For this review, take the finished solid that the model builds, in its own axes (mm). A direction names the side the tool comes from. Round coordinates to 2 decimals unless told otherwise and drop trailing zeros. Write each loop counter-clockwise with the first axis right and the second up, starting at its lowest first coordinate (ties: lowest second). Pieces come first, ordered by that corner, then holes.
Solid Edge part; units mm, degrees
sketch "Sketch1" plane through (0, 0, 0) normal (0, -1, 0) x (1, 0, 0)
  circle A0 centre (0, 0) radius 4.5
extrude "Protrusion1" add sketch "Sketch1" against normal blind 170
hole "Hole_1" at (0, 3, 0) direction (-1, 0, 0) diameter 3 end up to next
hole "Hole_4" at (0, 164, 0) direction (1, 0, 0) diameter 7.94 end up to next
(1) We need section C-C, the plane y = 3. Give the boundary of the cut face in (x, z), and give its area (3 significant figures).
Geometry check:
outline: (-4.24, -1.5) arc R4.5 ccw (long way) to (-4.24, 1.5) - (0, 1.5) - (0, -1.5) - close
area: 50.4 mm2
(2) We need section D-D, the plane y = 164. Give the boundary of the cut face in (x, z), and give its area (3 significant figures).
Geometry check:
outline: (0, -3.97) - (0, 3.97) - (2.12, 3.97) arc R4.5 ccw (long way) to (2.12, -3.97) - close
area: 33.3 mm2
(3) We need section B-B, the plane y = 114. Give the boundary of the cut face in (x, z), and give its area (3 significant figures).
Geometry check:
outline: circle Ø9 at (0, 0)
area: 63.6 mm2
(4) We need section A-A, the plane z = 0. Give the boundary of the cut face in (x, y), and give its area (3 significant figures).
Geometry check:
outline: (-4.5, 0) - (4.5, 0) - (4.5, 160.03) - (0, 160.03) - (0, 167.97) - (4.5, 167.97) - (4.5, 170) - (-4.5, 170) - (-4.5, 4.5) - (0, 4.5) - (0, 1.5) - (-4.5, 1.5) - close
area: 1,480 mm2
(5) For pin 1 Ø4 at (y, z) = (163.5, -0.5) entering from +X; pin 2 Ø3 at (x, y) = (3, 104) entering from +Z; pin 3 Ø5 at (x, y) = (3, 107.5) entering from +Z, all flat-tipped, find the tip position at first contact; note any pin that passes through.
Geometry check:
pin 1: stops at x = 0
pin 2: stops at z = 4.24
pin 3: stops at z = 4.47
(6) For faces 1 (the face through (-0.59, 83.81, 4.46)), 2 (the face through (-2.219, 1.536, 0.325)), 3 (the face through (0, 164, 0)), list the 3-axis set-ups (+Z, -Z, +X, -X, +Y, -Y) from which the entire face can be reached by the end or side of a thin tool; tool diameter is ignored.
Geometry check:
face 1: +Y, -Y
face 2: -X
face 3: +X
(7) For line 1 along Y through (x, z) = (1.2, 0); line 2 along Y through (x, z) = (-1, 0); line 3 along Z through (x, y) = (0.5, 57.5), list the stretches that pass through material, from the lowest coordinate up.
Geometry check:
line 1: y = 0 to 160.03, 167.97 to 170
line 2: y = 0 to 1.5, 4.5 to 170
line 3: z = -4.47 to 4.47
(8) Mouldability with a two-part tool opening along Y and no side actions: class faces 4 (the face through (0, 3, 0)), 5 (the face through (1.72, 167.35, 2.13)), 6 (the face through (0, 170, 0)), 7 (the face through (0, 0, 0)) as pulls with the +Y half, pulls with the -Y half, needs draft (parallel to the pull), parting line crosses it, or undercut.
Geometry check:
face 4: undercut
face 5: undercut
face 6: pulls with the +Y half
face 7: pulls with the -Y half
